from build123d import *

# Parameters (mm, degrees)
SKETCH_1_W            = 37
SKETCH_1_H            = 32
EXTRUDE_1_DEPTH       = 1.6
SKETCH_2_W            = 6.5
SKETCH_2_H            = 5
CUT_EXTRUDE_1_DEPTH   = 25.511425907
FILLET_1_R            = 2
HOLE_WIZARD_M31_D     = 3.4
HOLE_WIZARD_M31_DEPTH = 18
HOLE_WIZARD_M31_TIP   = 1.021463052
SKETCH_7_W            = 1.6
SKETCH_7_H            = 24.851674328
CUT_EXTRUDE_2_DEPTH   = 2


with BuildPart() as part:
    # Эскиз1 → Бобышка-Вытянуть1 (new body)
    with BuildSketch(Plane.XY):
        Rectangle(SKETCH_1_W, SKETCH_1_H)
    extrude(amount=EXTRUDE_1_DEPTH)

    # Эскиз2 → Вырез-Вытянуть1 (cut, through all)
    with BuildSketch(Plane.XY.offset(1.6)):
        with Locations((-15.25, 13.5)):
            Rectangle(SKETCH_2_W, SKETCH_2_H)
        with Locations((15.25, 13.5)):
            Rectangle(SKETCH_2_W, SKETCH_2_H)
        with Locations((15.25, -13.5)):
            Rectangle(SKETCH_2_W, SKETCH_2_H)
        with Locations((-15.25, -13.5)):
            Rectangle(SKETCH_2_W, SKETCH_2_H)
    extrude(amount=-CUT_EXTRUDE_1_DEPTH, mode=Mode.SUBTRACT)

    # Скругление1
    fillet_1_edges = [part.edges().sort_by_distance(p)[0] for p in [
        (-12, 11, 0.8),
        (12, 11, 0.8),
        (12, -11, 0.8),
        (-12, -11, 0.8),
    ]]
    fillet(fillet_1_edges, radius=FILLET_1_R)

    # Отверстие с зазором M31
    with Locations(Plane.XY.offset(1.6)):
        with Locations((-12.033502432, 7.1550555), (12.033502432, 7.1550555), (12.033502432, -7.1550555), (-12.033502432, -7.1550555)):
            Hole(HOLE_WIZARD_M31_D / 2, depth=HOLE_WIZARD_M31_DEPTH)
            with Locations((0, 0, -(HOLE_WIZARD_M31_DEPTH + HOLE_WIZARD_M31_TIP / 2))):  # 118° drill point
                Cone(0, HOLE_WIZARD_M31_D / 2, HOLE_WIZARD_M31_TIP, mode=Mode.SUBTRACT)

    # Эскиз7 → Вырез-Вытянуть2 (cut)
    with BuildSketch(Plane(origin=(18.5, 0, 0), x_dir=(0, 0, -1), z_dir=(1, 0, 0))):
        with Locations((-0.8, 0)):
            Rectangle(SKETCH_7_W, SKETCH_7_H)
    extrude(amount=-CUT_EXTRUDE_2_DEPTH, mode=Mode.SUBTRACT)


solid = part.part
Can you work these out from the model? Positions are in its coordinate system, mm. A direction names the side the tool comes from. Round coordinates to 2 decimals unless told otherwise and drop trailing zeros. Loops run counter-clockwise (first coordinate to the right, second up) from the corner with the lowest first, then second, coordinate; pieces in that order, holes last. Notation, with made-up numbers: (70.25, -20.75) - (124.25, -20.75) arc R20 cw to (124.25, 18.25) - close; hole circle Ø2 at (-17.5, -16). An arc over 180 degrees is marked (long way). Write item = value, one per line. Start each with the question number.
(1) If we section it at D-D (y = 8): Please give me the cut outline in (x, z).
(2) If we section it at A-A (y = -6): Please give me the cut outline in (x, z), and give its area (3 significant figures).
(3) If I drill on probe 1 along X at (y, z) = (6, 0.85); probe 2 along Y at (x, z) = (-13, 0.4); probe 3 along Y at (x, z) = (-16.5, 0.9), over which ranges is the centre line in solid material (lowest first)? Write a range as [from, to].
(4) For faces 4 (the face through (12, 14, 1)), 5 (the face through (-16, -11, 1)), 6 (the face through (-12, 14, 1)), which set-ups out of +Z, -Z, +X, -X, +Y, -Y let a thin tool reach every point of the face, with its end or its side?
(5) For P1, Ø4, axis at x = 12.03, y = 7.16, coming from the -Z side; P2, Ø0.5, axis at y = 15, z = 1, coming from the +X side; P3, Ø0.5, axis at x = 15.5, z = 0.5, coming from the -Y side, each with a flat end and sliding along its axis, tell me the tip position at first contact or that it passes through.
(6) If we mould it in two halves opening along X, with no side actions, what happens to faces 1 (the face through (11.249, -8.663, 0.789)), 2 (the face through (-16, 11, 1)), 3 (the face through (12.6, -11.57, 0.79))? For each: released by +X, released by -X, zero draft, split by the parting line, or undercut.
(7) If we section it at C-C (y = 13.5): Please give me the cut outline in (x, z), and give its area (3 significant figures).
(8) If we section it at B-B (z = 0.9): Please give me the cut outline in (x, y), and give its area (3 significant figures).
Ans:
q1.outline = (-18.5, 0) - (-13.51, 0) - (-13.51, 1.6) - (-18.5, 1.6) - close; (-10.56, 0) - (10.56, 0) - (10.56, 1.6) - (-10.56, 1.6) - close; (13.51, 0) - (16.5, 0) - (16.5, 1.6) - (13.51, 1.6) - close
q2.outline = (-18.5, 0) - (-13.28, 0) - (-13.28, 1.6) - (-18.5, 1.6) - close; (-10.79, 0) - (10.79, 0) - (10.79, 1.6) - (-10.79, 1.6) - close; (13.28, 0) - (16.5, 0) - (16.5, 1.6) - (13.28, 1.6) - close
q2.area = 48.0 mm²
q3.probe_1 = [-18.5, -13.28], [-10.79, 10.79], [13.28, 16.5]
q3.probe_2 = [-11.27, -8.55], [-5.76, 5.76], [8.55, 11.27]
q3.probe_3 = [-11, 11]
q4.face_4 = +Z, -Z, +X, +Y
q4.face_5 = +Z, -Z, -X, -Y
q4.face_6 = +Z, -Z, -X, +Y
q5.P1 = 0
q5.P2 = 12
q5.P3 = -11
q6.face_1 = undercut
q6.face_2 = zero draft
q6.face_3 = released by +X
q7.outline = (-12, 0) - (12, 0) - (12, 1.6) - (-12, 1.6) - close
q7.area = 38.4 mm²
q8.outline = (-18.5, -11) - (-14, -11) arc R2 cw to (-12, -13) - (-12, -16) - (12, -16) - (12, -13) arc R2 cw to (14, -11) - (16.5, -11) - (16.5, 11) - (14, 11) arc R2 cw to (12, 13) - (12, 16) - (-12, 16) - (-12, 13) arc R2 cw to (-14, 11) - (-18.5, 11) - close; hole circle Ø3.4 at (-12.03, -7.16); hole circle Ø3.4 at (-12.03, 7.16); hole circle Ø3.4 at (12.03, -7.16); hole circle Ø3.4 at (12.03, 7.16)
q8.area = 977 mm²
